The listing builds one solid part. Answer for the finished solid, in the listing's coordinates (mm). A direction names the side the tool comes from. Round coordinates to 2 decimals unless told otherwise and drop trailing zeros. Write each loop counter-clockwise with the first axis right and the second up, starting at its lowest first coordinate (ties: lowest second). Pieces come first, ordered by that corner, then holes. Notation, with made-up numbers: (16.25, 18) - (61.25, 18) arc R17 ccw to (61.25, 33) - close; hole circle Ø3 at (77.5, 9). An arc over 180 degrees is marked (long way). Use a Markdown table: item, result. Add a question column.
1) A tool of negligible diameter and unlimited length cuts with its end or side. For faces 4 (the flat face through (-1, 43, 150)), 5 (the cylindrical face through (-11.56, -8.62, -15.08)), 6 (the flat face through (0, 43, 0)), 7 (the flat face through (-1, -16, 150)), 8 (the flat face through (-1, -32, 323)), from which of +Z, -Z, +X, -X, +Y, -Y can it reach the whole face along a straight path? Write none if from no direction.
2) A cutting plane is placed at B-B (y = 37.5). Give the vertices of the cut face in (x, z), then the cut area to 3 significant figures.
3) A cutting plane is placed at A-A (x = 0). Give the vertices of the cut face in (y, z).
4) Each of these flat-tipped pins is pushed along its axis until it touches: P1, Ø1.5, axis at x = -18, y = -1.5, coming from the -Z side; P2, Ø4, axis at x = 13.5, y = 6.5, coming from the -Z side; P3, Ø8, axis at x = -42.5, y = -7, coming from the -Z side. Where does it stop, or does it pass through?
5) A cutting plane is placed at D-D (x = -51). Give the vertices of the cut face in (y, z), then the cut area to 3 significant figures.
6) Find the intervals of material crossed by probe 1 along Z at (x, y) = (36, -6.5); probe 2 along Y at (x, z) = (-31, 43.5); probe 3 along Z at (x, y) = (15.5, -10), in increasing order. Write a range as from..to.
7) Determine the mould class of faces 1 (the flat face through (0, -17, 0)), 2 (the flat face through (-1, 12, 500)), 3 (the cylindrical face through (-11.56, 35.39, -15.08)) for opening direction Z: +Z half, -Z half, draft (parallel to the pull), parting line (faces both ways), or undercut.
8) A cutting plane is placed at C-C (z = 0). Give the vertices of the cut face in (x, y), then the cut area to 3 significant figures.
```python
from build123d import *

# Parameters (mm, degrees)
SKETCH1_R                = 39.5
BOSS_EXTRUDE1_DEPTH      = 28
BOSS_EXTRUDE2_DEPTH      = 15
BOSS_EXTRUDE2_DEPTH_BACK = 45
SKETCH2_R                = 19
BOSS_EXTRUDE3_DEPTH      = 28
BOSS_EXTRUDE4_DEPTH      = 30
BOSS_EXTRUDE4_DEPTH_BACK = 60
SKETCH4_W                = 150
SKETCH4_H                = 350


with BuildPart() as part:
    # Sketch1 → Boss-Extrude1 (new body)
    with BuildSketch(Plane(origin=(0, 0, 0), x_dir=(1, 0, 0), z_dir=(0, 1, 0))):
        with Locations(Location((0, 0, 0), (0, 0, 270))):
            Circle(SKETCH1_R)
    extrude(amount=BOSS_EXTRUDE1_DEPTH)

    # Sketch2 → Boss-Extrude2 (add, two sides: drawn at the far end of the back side and taken through both)
    with BuildSketch(Plane(origin=(0, 28, 0), x_dir=(1, 0, 0), z_dir=(0, 1, 0)).offset(-BOSS_EXTRUDE2_DEPTH_BACK)):
        with Locations(Location((0, 0, 0), (0, 0, 270))):
            Circle(SKETCH2_R)
    extrude(amount=BOSS_EXTRUDE2_DEPTH + BOSS_EXTRUDE2_DEPTH_BACK)

    # Sketch3 → Boss-Extrude3 (add)
    with BuildSketch(Plane(origin=(0, 0, 0), x_dir=(1, 0, 0), z_dir=(0, 1, 0))):
        Polygon((0, 0), (-75, -50), (-75, -500), (75, -500), (75, -50), align=None)
    extrude(amount=BOSS_EXTRUDE3_DEPTH)

    # Sketch4 → Boss-Extrude4 (add, two sides: drawn at the far end of the back side and taken through both)
    with BuildSketch(Plane(origin=(0, 28, 0), x_dir=(1, 0, 0), z_dir=(0, 1, 0)).offset(-BOSS_EXTRUDE4_DEPTH_BACK)):
        with Locations((0, -325)):
            Rectangle(SKETCH4_W, SKETCH4_H)
    extrude(amount=BOSS_EXTRUDE4_DEPTH + BOSS_EXTRUDE4_DEPTH_BACK)


solid = part.part
```
Entries:
| question | item | result |
|---|---|---|
| 1 | face 4 | +X, -X, +Y |
| 1 | face 5 | -Y |
| 1 | face 6 | -Z, +X, -X, +Y |
| 1 | face 7 | +X, -X, -Y |
| 1 | face 8 | +Z, -Z, +X, -X, -Y |
| 2 | outline | (-75, 150) - (75, 150) - (75, 500) - (-75, 500) - close; circle Ø38 at (0, 0) |
| 2 | area | 53,600 mm² |
| 3 | outline | (-32, 150) - (0, 150) - (0, 19) - (-17, 19) - (-17, -19) - (0, -19) - (0, -39.5) - (28, -39.5) - (28, -19) - (43, -19) - (43, 19) - (28, 19) - (28, 150) - (58, 150) - (58, 500) - (-32, 500) - close |
| 4 | P1 | stops at z = -7.96 |
| 4 | P2 | stops at z = -37.79 |
| 4 | P3 | stops at z = 150 |
| 5 | outline | (-32, 150) - (0, 150) - (0, 34) - (28, 34) - (28, 150) - (58, 150) - (58, 500) - (-32, 500) - close |
| 5 | area | 34,700 mm² |
| 6 | probe 1 | z = 150..500 |
| 6 | probe 2 | y = 0..28 |
| 6 | probe 3 | z = -10.99..10.99, 150..500 |
| 7 | face 1 | draft |
| 7 | face 2 | +Z half |
| 7 | face 3 | undercut |
| 8 | outline | (-39.5, 0) - (-19, 0) - (-19, -17) - (19, -17) - (19, 0) - (39.5, 0) - (39.5, 28) - (19, 28) - (19, 43) - (-19, 43) - (-19, 28) - (-39.5, 28) - close |
| 8 | area | 3,430 mm² |
